Build history of the part. All positions in model axes, mm. Face numbers are marked on the shaded views. A direction names the side the tool comes from. Give positions to 0.01 mm unless a question says otherwise; leave off trailing zeros. Order: outer loops, then holes, each group sorted by start corner. A loop starts at its lowest first (then second) coordinate and runs counter-clockwise, first axis right, second up. Notation, with made-up numbers: (28, 57) - (78, 57) arc R15 ccw to (78, 63) - close; hole circle Ø2 at (56.5, 18). An arc over 180 degrees is marked (long way). One line per item, written item: value.
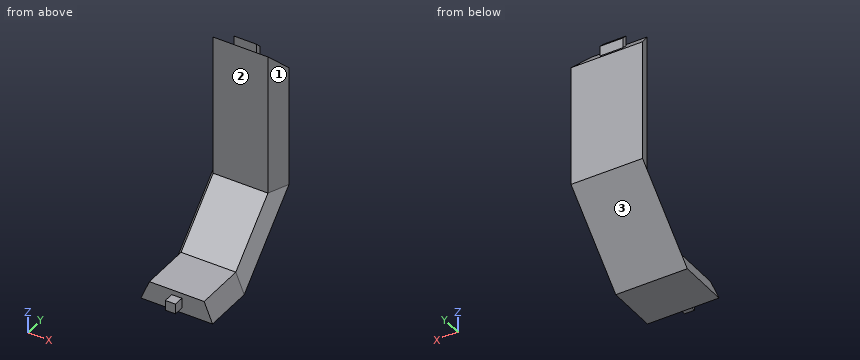
```python
from build123d import *

# Parameters (mm, degrees)
BOSS_EXTRUDE1_DEPTH     = 10
BOSS_EXTRUDE5_DEPTH     = 20
CUT_EXTRUDE1_DEPTH      = 43.284970512
CUT_EXTRUDE1_DEPTH_BACK = 43.284970512
BOSS_EXTRUDE7_DEPTH     = 28
CUT_EXTRUDE3_DEPTH      = 52.790286451
CUT_EXTRUDE3_DEPTH_BACK = 52.790286451
SKETCH31_W              = 4.5
SKETCH31_H              = 1.5
BOSS_EXTRUDE8_DEPTH     = 2
SKETCH32_W              = 2
SKETCH32_H              = 2
BOSS_EXTRUDE9_DEPTH     = 2


with BuildPart() as part:
    # Sketch2 → Boss-Extrude1 (new body)
    with BuildSketch(Plane(origin=(0, 0, 0), x_dir=(1, 0, 0), z_dir=(0, 1, 0))):
        Polygon((30.067911316, 5.900626551), (31.724765565, 1.900626551), (42.55319269, 1.900626551), (44.21004694, 5.900626551), align=None)
    extrude(amount=BOSS_EXTRUDE1_DEPTH)

    # Sketch9 → Boss-Extrude5 (add, along a direction that is not the sketch's normal)
    with BuildSketch(Plane(origin=(0, 10, 0), x_dir=(1, 0, 0), z_dir=(0, 1, 0))):
        Polygon((30.067911316, 5.900626551), (31.724765565, 1.900626551), (42.55319269, 1.900626551), (44.21004694, 5.900626551), align=None)
    extrude(amount=BOSS_EXTRUDE5_DEPTH, dir=(1.7578001538897393e-15, 0.7071067811865437, 0.7071067811865515))

    # Sketch14 → Cut-Extrude1 (cut, two sides: drawn at the far end of the back side and taken through both)
    with BuildSketch(Plane(origin=(37.138979128, -13.011121517, 13.011121517), x_dir=(-2.5975542964999143e-15, -0.11094714299783787, -0.9938263084969211), z_dir=(1, 0, 0)).offset(-CUT_EXTRUDE1_DEPTH_BACK)):
        Polygon((0.618118596, 37.453059267), (-3.357186638, 37.009270695), (1.061907168, 33.477754033), align=None)
    extrude(amount=CUT_EXTRUDE1_DEPTH + CUT_EXTRUDE1_DEPTH_BACK, mode=Mode.SUBTRACT)

    # Sketch15 → Boss-Extrude7 (add)
    with BuildSketch(Plane.XY.offset(8.241509073)):
        Polygon((30.067911316, 24.142135624), (31.724765565, 20.142135624), (42.55319269, 20.142135624), (44.21004694, 24.142135624), align=None)
    extrude(amount=BOSS_EXTRUDE7_DEPTH)

    # Sketch30 → Cut-Extrude3 (cut, two sides: drawn at the far end of the back side and taken through both)
    with BuildSketch(Plane(origin=(37.138979128, -12.611751667, 0.445063165), x_dir=(-2.6136735802757005e-15, -0.0035891178684094257, -0.9999935590957207), z_dir=(1, 0, 0)).offset(-CUT_EXTRUDE3_DEPTH_BACK)):
        Polygon((-35.928129381, 36.625172899), (-35.913772909, 32.625198662), (-31.928155144, 36.63952937), align=None)
    extrude(amount=CUT_EXTRUDE3_DEPTH + CUT_EXTRUDE3_DEPTH_BACK, mode=Mode.SUBTRACT)

    # Sketch31 → Boss-Extrude8 (add, along a direction that is not the sketch's normal)
    with BuildSketch(Plane(origin=(0, 28.191822348, 28.191822348), x_dir=(1, 0, 0), z_dir=(0, 0.7071067811865434, 0.7071067811865517))):
        with Locations((37.138979128, -8.555549014)):
            Rectangle(SKETCH31_W, SKETCH31_H)
    extrude(amount=BOSS_EXTRUDE8_DEPTH, dir=(0, 0, 1))

    # Sketch32 → Boss-Extrude9 (add)
    with BuildSketch(Plane.XZ):
        with Locations((37.138979128, -3.900626551)):
            Rectangle(SKETCH32_W, SKETCH32_H)
    extrude(amount=BOSS_EXTRUDE9_DEPTH)


solid = part.part
```
(1) 3-axis set-ups, long thin cutter, end or side, ignore diameter. For the marked faces 1, 2 and 3: which of +Z, -Z, +X, -X, +Y, -Y reach the whole face in a straight line?
Completed:
face 1: +Z, +X, -Y
face 2: +Z, +X, -X, -Y
face 3: -Z, +X, -X, +Y
(2) Slice it at B-B, the plane z = 10. Give the cut face in (x, y), and give its area (3 significant figures).
Completed:
outline: (30.07, 24.14) - (31.72, 20.14) - (42.55, 20.14) - (44.21, 24.14) - close
area: 49.9 mm²
(3) Slice it at C-C, the plane x = 37. Give the cut face in (y, z), and give its area (3 significant figures).
Completed:
outline: (-2, -4.9) - (0, -4.9) - (0, -5.9) - (10, -5.9) - (24.14, 8.24) - (24.14, 32.24) - (22.67, 33.71) - (22.67, 35.71) - (21.61, 36.77) - (21.61, 34.77) - (20.14, 36.24) - (20.14, 8.24) - (10, -1.9) - (0, -1.9) - (0, -2.9) - (-2, -2.9) - close
area: 199 mm²
(4) Drill centre lines: line 1 (Y direction, x = 33.5, z = 15); line 2 (Z direction, x = 39.75, y = 9.5); line 3 (Z direction, x = 43, y = 4.5). Where is each one in solid material? Low to high.
Completed:
line 1: 20.14 to 24.14
line 2: -5.9 to -1.9
line 3: -5.9 to -2.98
(5) Pin check, flat tips, straight feed: P1, Ø3, axis at x = 34.5, z = 23, coming from the -Y side; P2, Ø1.6, axis at x = 37, y = -1, coming from the -Z side; P3, Ø12, axis at y = 16.5, z = 20, coming from the +X side. Stop position of each tip, or through.
Completed:
P1: y = 20.14
P2: z = -4.9
P3: x = 43.53
(6) Slice it at D-D, the plane y = 6.25. Give the cut face in (x, z), and give its area (3 significant figures).
Completed:
outline: (30.07, -5.9) - (44.21, -5.9) - (42.55, -1.9) - (31.72, -1.9) - close
area: 49.9 mm²
(7) Slice it at A-A, the plane x = 40.25. Give the cut face in (y, z).
Completed:
outline: (0, -5.9) - (10, -5.9) - (24.14, 8.24) - (24.14, 32.24) - (20.14, 36.24) - (20.14, 8.24) - (10, -1.9) - (0, -1.9) - close
